Read the model definition and answer for the solid it produces. Units are mm, in the model's axes. A direction names the side the tool comes from. Coordinates: 2 decimals unless noted, no trailing zeros. Loops run counter-clockwise (first coordinate to the right, second up) from the corner with the lowest first, then second, coordinate; pieces in that order, holes last. Notation, with made-up numbers: M -22.5,5.5 L 33.5,5.5 A14 cw 33.5,21.5 Z; hole C 1.25,50.5 d1. An arc over 180 degrees is marked long. Use one line per item in the form item = value. Start each with the question number.
1. A tool of negligible diameter and unlimited length cuts with its end or side. For faces 5 (the flat face through (0, -10, 9)), 6 (the cylindrical face through (6.6, 13.38, 14.14)), 7 (the flat face through (-5.5, 20, 0)), 8 (the flat face through (-7.5, 20, 0)), 9 (the flat face through (5.5, 20, 7)), from which of +Z, -Z, +X, -X, +Y, -Y can it reach the whole face along a straight path? Write none if from no direction.
2. The part is cut by section A-A (z = -7.75). Give the vertices of the cut face in (x, y).
3. The part is cut by section B-B (y = 25.5). Give the number of separate pieces and of enclosed holes in the cut face, plus the area to 3 significant figures.
4. For a pull along X with two mould halves and no side action, classify faces 1 (the cylindrical face through (-5.361, -17.745, -10.479)), 2 (the flat face through (6, 0, 0)), 3 (the flat face through (3, 20, -4)), 4 (the flat face through (-5, 20, 2)) as released by +X, released by -X, zero draft, split by the parting line, or undercut.
5. Find the intervals of material crossed by probe 1 along Z at (x, y) = (-2.25, 28); probe 2 along X at (y, z) = (26.5, 0.5); probe 3 along X at (y, z) = (8.5, 7), in increasing order. Write a range as [from, to].
6. Flat-ended cylindrical pins translate along their axes: pin 1 (3 mm diameter, centred on x = 4.5, z = 2, fed in from -Y); pin 2 (6 mm diameter, centred on x = 0, z = -6, fed in from +Y). Find the tip coordinate at first contact, or state that the pin passes through.
from build123d import *

# Parameters (mm, degrees)
SKETCH1_W           = 15
SKETCH1_H           = 30
SKETCH1_W_2         = 2
SKETCH1_H_2         = 4
BOSS_EXTRUDE1_DEPTH = 40
SKETCH2_W           = 15
SKETCH2_H           = 6
BOSS_EXTRUDE2_DEPTH = 20
FILLET1_R           = 7.5
SKETCH3_R           = 1.5
CUT_EXTRUDE1_DEPTH  = 51.55937104
FILLET2_R           = 3


with BuildPart() as part:
    # Sketch1 → Boss-Extrude1 (new body)
    with BuildSketch(Plane(origin=(0, 0, 0), x_dir=(1, 0, 0), z_dir=(0, 1, 0))):
        Rectangle(SKETCH1_W, SKETCH1_H)
        Polygon((-5.5, -13), (5.5, -13), (5.5, -4), (1.5, -4), (1.5, 4), (5.5, 4), (5.5, 13), (-5.5, 13), (-5.5, 4), (-1.5, 4), (-1.5, -4), (-5.5, -4), align=None, mode=Mode.SUBTRACT)
        with Locations((-4.5, 0)):
            Rectangle(SKETCH1_W_2, SKETCH1_H_2, mode=Mode.SUBTRACT)
        with Locations((4.5, 0)):
            Rectangle(SKETCH1_W_2, SKETCH1_H_2, mode=Mode.SUBTRACT)
    extrude(amount=BOSS_EXTRUDE1_DEPTH)

    # Sketch2 → Boss-Extrude2 (add)
    with BuildSketch(Plane.XZ):
        with Locations((0, 12)):
            Rectangle(SKETCH2_W, SKETCH2_H)
        with Locations((0, -12)):
            Rectangle(SKETCH2_W, SKETCH2_H)
    extrude(amount=BOSS_EXTRUDE2_DEPTH)

    # Fillet1
    fillet1_edges = [part.edges().sort_by_distance(p)[0] for p in [
        (-7.5, -20, 12),
        (-7.5, -20, -12),
        (7.5, -20, -12),
        (7.5, -20, 12),
    ]]
    fillet(fillet1_edges, radius=FILLET1_R - 0.0001)  # a hair under: the kernel refuses the full size

    # Sketch3 → Cut-Extrude1 (cut, through all)
    with BuildSketch(Plane.XY.offset(15)):
        with Locations((0, -12.5)):
            Circle(SKETCH3_R)
    extrude(amount=-CUT_EXTRUDE1_DEPTH, mode=Mode.SUBTRACT)

    # Fillet2
    fillet2_edges = [part.edges().sort_by_distance(p)[0] for p in [
        (5.303330148, -17.803330148, 15),
        (-5.303330148, -17.803330148, 15),
        (5.303330148, -17.803330148, -15),
        (-5.303330148, -17.803330148, -15),
        (5.5, 20, -13),
        (-5.5, 20, -13),
        (-5.5, 20, 13),
        (5.5, 20, 13),
        (7.5, 13.74995, 15),
        (-7.5, 13.74995, 15),
        (-7.5, 13.74995, -15),
        (7.5, 13.74995, -15),
    ]]
    fillet(fillet2_edges, radius=FILLET2_R)


solid = part.part
Computed values:
q1.face_5 = +X, -X, -Y
q1.face_6 = +Z, +X, +Y, -Y
q1.face_7 = +Y, -Y
q1.face_8 = +Z, -Z, -X, +Y, -Y
q1.face_9 = +Y
q2.outline = M -7.5,0 L -5.5,0 L -5.5,40 L -7.5,40 Z; M 5.5,0 L 7.5,0 L 7.5,40 L 5.5,40 Z
q3.separate_pieces = 1
q3.enclosed_holes = 3
q3.area = 212 mm²
q4.face_1 = released by -X
q4.face_2 = zero draft
q4.face_3 = undercut
q4.face_4 = undercut
q5.probe_1 = [-15, -13], [-4, 4], [13, 15]
q5.probe_2 = [-7.5, -5.5], [-3.5, -1.5], [1.5, 3.5], [5.5, 7.5]
q5.probe_3 = [-7.5, -5.5], [5.5, 7.5]
q6.pin_1 = 0
q6.pin_2 = 40
